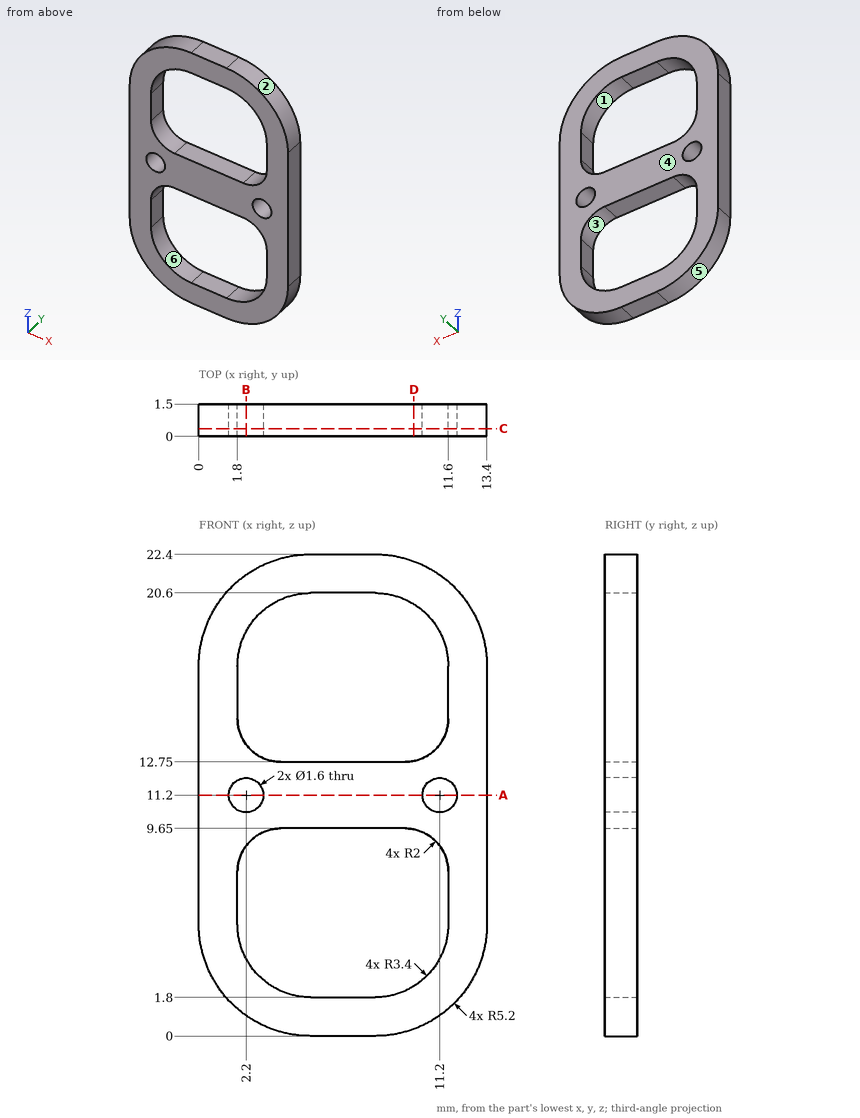
Drawing for the job (mm, zero at the part's lowest x, y, z). A direction names the side the tool comes from. Give positions to 0.01 mm unless a question says otherwise; leave off trailing zeros. Order: outer loops, then holes, each group sorted by start corner. A loop starts at its lowest first (then second) coordinate and runs counter-clockwise, first axis right, second up. Notation, with made-up numbers: (-14.5, 27) - (1.5, 27) arc R26 cw to (1.5, 51) - close; hole circle Ø8 at (8, -19.75). An arc over 180 degrees is marked (long way). Write item = value, one per line. Start each with the question number.
1. Cut at C-C, the plane y = 0.35. List the corners of the cut face in (x, z).
2. Two-plate mould, pull along X, no slides. Class the marked faces 1, 2, 3 and 4: pulls with the +X half, pulls with the -X half, needs draft (parallel to the pull), parting line crosses it, or undercut.
3. Cut at D-D, the plane x = 10. List the corners of the cut face in (y, z) (1 decimal).
4. Which spindle directions (+Z, -Z, +X, -X, +Y, -Y) get a long thin tool onto all of the face, cutting with end or side? Do the marked faces 5 and 6. Say none if no direction does.
5. Cut at A-A, the plane z = 11.2. List the corners of the cut face in (x, y), and give its area (3 significant figures).
6. Probe line 1 along X through (y, z) = (0.25, 15.5); line 2 along Z through (x, y) = (6.5, 0.65); line 3 along Z through (x, y) = (4, 0.1). List the from-to ranges inside material, lowest first.
7. Cut at B-B, the plane x = 2.2. List the corners of the cut face in (y, z), and give its area (3 significant figures).
Taken from the geometry:
q1.outline = (0, 5.2) arc R5.2 ccw to (5.2, 0) - (8.2, 0) arc R5.2 ccw to (13.4, 5.2) - (13.4, 17.2) arc R5.2 ccw to (8.2, 22.4) - (5.2, 22.4) arc R5.2 ccw to (0, 17.2) - close; hole circle Ø1.6 at (2.2, 11.2); hole (1.8, 5.2) arc R3.4 ccw to (5.2, 1.8) - (8.2, 1.8) arc R3.4 ccw to (11.6, 5.2) - (11.6, 7.65) arc R2 ccw to (9.6, 9.65) - (3.8, 9.65) arc R2 ccw to (1.8, 7.65) - close; hole (1.8, 14.75) arc R2 ccw to (3.8, 12.75) - (9.6, 12.75) arc R2 ccw to (11.6, 14.75) - (11.6, 17.2) arc R3.4 ccw to (8.2, 20.6) - (5.2, 20.6) arc R3.4 ccw to (1.8, 17.2) - close; hole circle Ø1.6 at (11.2, 11.2)
q2.face_1 = undercut
q2.face_2 = pulls with the +X half
q2.face_3 = undercut
q2.face_4 = needs draft
q3.outline = (0, 0.3) - (1.5, 0.3) - (1.5, 2.3) - (0, 2.3) - close; (0, 9.6) - (1.5, 9.6) - (1.5, 12.8) - (0, 12.8) - close; (0, 20.1) - (1.5, 20.1) - (1.5, 22.1) - (0, 22.1) - close
q4.face_5 = -Z, -X, +Y, -Y
q4.face_6 = +Y, -Y
q5.outline = (0, 0) - (1.4, 0) - (1.4, 1.5) - (0, 1.5) - close; (3, 0) - (10.4, 0) - (10.4, 1.5) - (3, 1.5) - close; (12, 0) - (13.4, 0) - (13.4, 1.5) - (12, 1.5) - close
q5.area = 15.3 mm²
q6.line_1 = 0 to 1.8, 11.6 to 13.4
q6.line_2 = 0 to 1.8, 9.65 to 12.75, 20.6 to 22.4
q6.line_3 = 0.14 to 2.02, 9.65 to 12.75, 20.38 to 22.26
q7.outline = (0, 0.95) - (1.5, 0.95) - (1.5, 3.6) - (0, 3.6) - close; (0, 8.85) - (1.5, 8.85) - (1.5, 10.4) - (0, 10.4) - close; (0, 12) - (1.5, 12) - (1.5, 13.55) - (0, 13.55) - close; (0, 18.8) - (1.5, 18.8) - (1.5, 21.45) - (0, 21.45) - close
q7.area = 12.6 mm²
